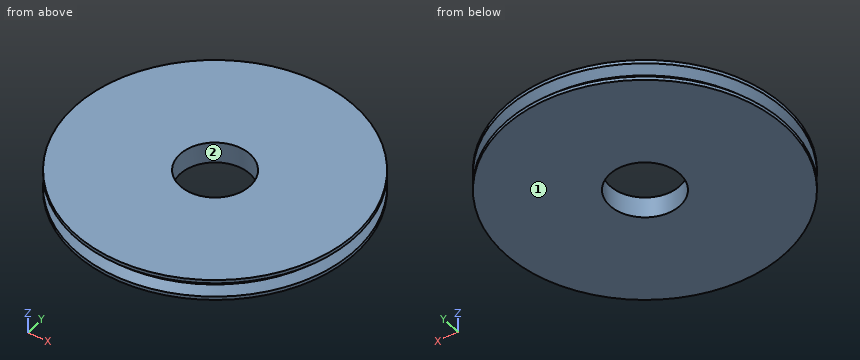
Autodesk Inventor part; units mm, degrees
ref_plane "YZ Plane" through (0, 0, 0) normal (1, 0, 0) x (0, 1, 0)
ref_plane "XZ Plane" through (0, 0, 0) normal (0, 1, 0) x (-1, 0, 0)
ref_plane "XY Plane" through (0, 0, 0) normal (0, 0, 1) x (1, 0, 0)
sketch "Sketch1" plane through (0, 0, 0) normal (0, 1, 0) x (-1, 0, 0)
  line L0 (9.5, 0.1897) -> (10, 0.6897)
  line L1 (10, 0.6897) -> (10, 0.9397)
  line L2 (10, 0.9397) -> (0, 0.9397)
  line L3 (9.5, 0.1897) -> (-0.1607, 0.1897) construction
  line L4 (9.5, 0.1897) -> (10, -0.3103)
  line L5 (10, -0.3103) -> (10, -0.5603)
  line L6 (10, -0.5603) -> (0, -0.5603)
  line L7 (0, 0.9397) -> (0, -0.5603)
  dimension "d1" = 1.5
  dimension "d2" = 1
  dimension "d3" = 90
revolve "Revolution1" add sketch "Sketch1" angle 360 about axis through (0, 0, 0.9397) along (0, 0, -1)
sketch "Sketch2" plane through (0, 0, -0.5603) normal (0, 0, -1) x (-1, 0, 0)
  circle A0 centre (0, 0) radius 10
  circle A1 centre (0, 0) radius 2.5
  point P0 (0, 0)
  dimension "d5" = 5
extrude "Extrusion1" cut sketch "Sketch2" against normal blind 10 contours A1
properties part number "kladicka"
Work out the finished part from the listing and answer in its coordinate system (mm). Face numbers are marked on the shaded views. Give positions to 0.01 mm unless a question says otherwise; leave off trailing zeros. Write each loop counter-clockwise with the first axis right and the second up, starting at its lowest first coordinate (ties: lowest second). Pieces come first, ordered by that corner, then holes.
Q1. For a pull along X with two mould halves and no side action, classify the marked faces 1 and 2 as released by +X, released by -X, zero draft, split by the parting line, or undercut.
Answer:
face 1: zero draft
face 2: undercut
Q2. The part is cut by section A-A on x = 0. Give the vertices of the cut face in (y, z), and give its area (3 significant figures).
Answer:
outline: (-10, -0.56) - (-2.5, -0.56) - (-2.5, 0.94) - (-10, 0.94) - (-10, 0.69) - (-9.5, 0.19) - (-10, -0.31) - close; (2.5, -0.56) - (10, -0.56) - (10, -0.31) - (9.5, 0.19) - (10, 0.69) - (10, 0.94) - (2.5, 0.94) - close
area: 22.0 mm2
Q3. Given pin 1 (8 mm diameter, centred on x = -1.5, y = -1, fed in from +Z); pin 2 (4 mm diameter, centred on x = 0, y = 0, fed in from +Z), each flat-ended and moving along its own axis, determine where each tip first touches the part or whether it passes through.
Answer:
pin 1: stops at z = 0.94
pin 2: passes through
Q4. Straight lines are drawn through the part: L1, parallel to X at y = -2.25, z = 0.9; L2, parallel to Y at x = 1, z = -0.45; L3, parallel to Y at x = 0, z = -0.05. For each, find the intervals that lie inside material, in ascending order.
Answer:
L1: x = -9.74 to -1.09, 1.09 to 9.74
L2: y = -9.95 to -2.29, 2.29 to 9.95
L3: y = -9.74 to -2.5, 2.5 to 9.74
